```python
from build123d import *

# Parameters (mm, degrees)
F0_R     = 15.875
F1_DEPTH = 6.35
F3_D     = 3.302
F4_R     = 3.17499


# Not quite as in the source:
# - a fillet or chamfer is up to 0.001 mm smaller than in the source, because OpenCascade refuses the exact size


with BuildPart() as f1:
    # F0 (on Front) → F1 (new body)
    with BuildSketch(Plane.XZ):
        Circle(F0_R)
    extrude(amount=F1_DEPTH)

    # F3 (through all)
    with Locations(Plane.XZ.offset(6.35)):
        with Locations((0, 0)):
            Hole(F3_D / 2)

    # F4 (radius 3.175 in the source; OpenCascade refuses exactly that, so slightly less here)
    f4_edges = [f1.edges().sort_by_distance(p)[0] for p in [
        (-15.875, -6.35, 0),
        (-15.875, 0, 0),
    ]]
    fillet(f4_edges, radius=F4_R)


solid = f1.part
```
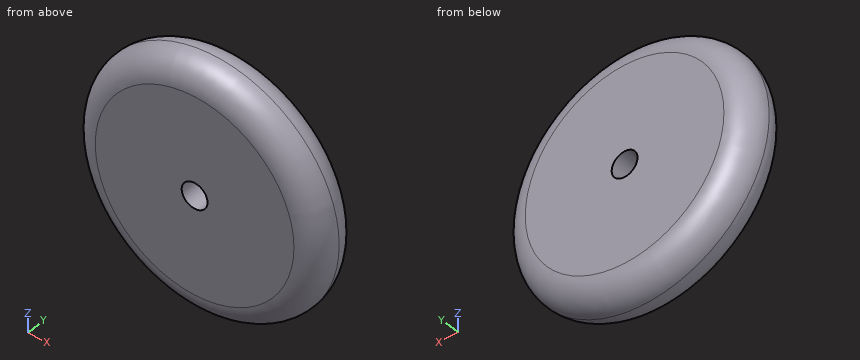
The listing builds one solid part. Answer for the finished solid, in the listing's coordinates (mm). Round coordinates to 2 decimals unless told otherwise and drop trailing zeros. Order: outer loops, then holes, each group sorted by start corner. A loop starts at its lowest first (then second) coordinate and runs counter-clockwise, first axis right, second up. Notation, with made-up numbers: (-16, 53.25) - (-4, 53.25) arc R21 cw to (-4, 59.25) - close; hole circle Ø9 at (-19, 49). An arc over 180 degrees is marked (long way). Put each result on its own line as item: value. Start each with the question number.
(1) Straight lines are drawn through the part: probe 1 along Z at (x, y) = (0, -2.5); probe 2 along Y at (x, z) = (-8, 10); probe 3 along Z at (x, y) = (0, -2.25). For each, find the intervals that lie inside material, in ascending order. Write a range as from..to.
(2) Given P1, Ø2, axis at x = 3, y = -1.5, coming from the +Z side; P2, Ø1, axis at y = -4, z = 5, coming from the +X side; P3, Ø4, axis at x = -10, z = -12.5, coming from the +Y side, each flat-ended and moving along its own axis, determine where each tip first touches the part or whether it passes through.
(3) Find section C-C (y = -1.75). Give the vertices of the cut face in (x, z).
(4) Find section B-B (y = -4). Give the vertices of the cut face in (x, z).
Reply:
1. probe 1: -15.8..-1.65, 1.65..15.8
1. probe 2: -6.35..0
1. probe 3: -15.74..-1.65, 1.65..15.74
2. P1: z = 15.57
2. P2: x = 15.15
2. P3: y = -0.28
3. outline: circle Ø31.07 at (0, 0); hole circle Ø3.3 at (0, 0)
4. outline: circle Ø31.53 at (0, 0); hole circle Ø3.3 at (0, 0)
